For this review, take the finished solid that the model builds, in its own axes (mm). A direction names the side the tool comes from. Round coordinates to 2 decimals unless told otherwise and drop trailing zeros. Write each loop counter-clockwise with the first axis right and the second up, starting at its lowest first coordinate (ties: lowest second). Pieces come first, ordered by that corner, then holes. Notation, with made-up numbers: (32.5, 50) -> (76.5, 50) arc R21 ccw to (76.5, 81) -> close; hole circle Ø2 at (52, -37). An arc over 180 degrees is marked (long way). Answer as CSV lines item,"result". Start each with the question number.
Item 1: Wall thickness on probe 1 along Y at (x, z) = (3, -2.75); probe 2 along X at (y, z) = (42, -1.75); probe 3 along Z at (x, y) = (-1, 43.5): over which ranges is each line inside the solid? List them lowest first. Write a range as from..to.
Item 2: Machinability: for faces 1 (the flat face through (0, 0, 0)), 2 (the cylindrical face through (0.9, 24.69, 2.86)), which of the approach directions +Z, -Z, +X, -X, +Y, -Y give a long, thin tool a straight path to every point of the face, cutting with its end or side? Answer none if there is none.
Item 3: Take a section at A-A on y = 5.5. Give the boundary of the cut face in (x, z).
Item 4: For pin 1 Ø1.5 at (y, z) = (17, -2.5) entering from +X; pin 2 Ø1.5 at (x, y) = (-2, 13) entering from -Z; pin 3 Ø2 at (x, y) = (3.5, 19.5) entering from -Z; pin 4 Ø5 at (x, z) = (-0.5, -1) entering from +Y, all flat-tipped, find the tip position at first contact; note any pin that passes through.
```python
from build123d import *

# Parameters (mm, degrees)
SKETCH1_R           = 6
SKETCH1_R_2         = 3
BOSS_EXTRUDE1_DEPTH = 3
SKETCH1_2_R         = 3
BOSS_EXTRUDE2_DEPTH = 50
CHAMFER1_SIZE       = 3


with BuildPart() as part:
    # Sketch1 → Boss-Extrude1 (new body)
    with BuildSketch(Plane(origin=(0, 0, 0), x_dir=(1, 0, 0), z_dir=(0, 1, 0))):
        with Locations(Location((0, 0, 0), (0, 0, 270))):
            Circle(SKETCH1_R)
        with Locations(Location((0, 0, 0), (0, 0, 270))):
            Circle(SKETCH1_R_2, mode=Mode.SUBTRACT)
    extrude(amount=BOSS_EXTRUDE1_DEPTH)

    # Sketch1<2> → Boss-Extrude2 (add)
    with BuildSketch(Plane(origin=(0, 0, 0), x_dir=(1, 0, 0), z_dir=(0, 1, 0))):
        with Locations(Location((0, 0, 0), (0, 0, 270))):
            Circle(SKETCH1_2_R)
    extrude(amount=BOSS_EXTRUDE2_DEPTH)

    # Chamfer1
    chamfer1_edges = [part.edges().sort_by_distance(p)[0] for p in [
        (0, 50, -3),
        (0, 3, -6),
    ]]
    chamfer(chamfer1_edges, length=CHAMFER1_SIZE - 0.0001)  # a hair under: the kernel refuses the full size


solid = part.part
```
Output values:
1,probe 1,"y = 0..1.93"
1,probe 2,"x = -2.44..2.44"
1,probe 3,"z = -2.83..2.83"
2,face 1,"+Z, -Z, +X, -X, -Y"
2,face 2,"+Y"
3,outline,"circle Ø6 at (0, 0)"
4,pin 1,"stops at x = 2.44"
4,pin 2,"stops at z = -2.73"
4,pin 3,"stops at z = -1.66"
4,pin 4,"stops at y = 50"
